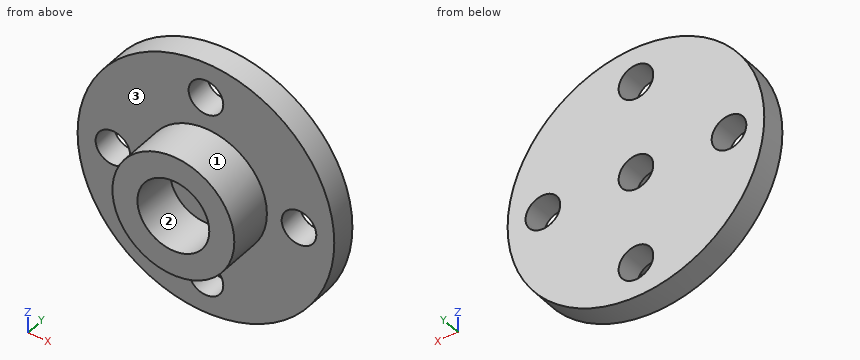
```python
from build123d import *

# Parameters (mm, degrees)
F0_R     = 10
F1_DEPTH = 2
F2_R     = 4.75
F2_R_2   = 2.8
F3_DEPTH = 3.6
F4_R     = 1.35
F5_DEPTH = 25


with BuildPart() as f1:
    # F0 (on Front) → F1 (new body)
    with BuildSketch(Plane.XZ):
        Circle(F0_R)
    extrude(amount=F1_DEPTH)

    # F2 (on face) → F3 (join)
    with BuildSketch(Plane.XZ.offset(2)):
        Circle(F2_R)
        Circle(F2_R_2, mode=Mode.SUBTRACT)
    extrude(amount=F3_DEPTH)

    # F4 (on face) → F5 (cut)
    with BuildSketch(Plane.XZ.offset(2)):
        with Locations((0, 7.25)):
            Circle(F4_R)
        with Locations((-7.25, 0)):
            Circle(F4_R)
        Circle(F4_R)
        with Locations((7.25, 0)):
            Circle(F4_R)
        with Locations((0, -7.25)):
            Circle(F4_R)
    extrude(amount=-F5_DEPTH, mode=Mode.SUBTRACT)


solid = f1.part
```
Source: CAD feature listing. Evaluate the final solid. Frame: model axes, mm. Face numbers are marked on the shaded views. Round coordinates to 2 decimals unless told otherwise and drop trailing zeros. Loops run counter-clockwise (first coordinate to the right, second up) from the corner with the lowest first, then second, coordinate; pieces in that order, holes last. Notation, with made-up numbers: M -2,36 L 20,36 A32 ccw 20,70 Z; hole C -27.75,84.25 d1. An arc over 180 degrees is marked long. Use a Markdown table: item, result. Add a question column.
1. Mould query, pull axis X, two halves, no side actions, for the marked faces 1, 2 and 3. Classes: pulls with the +X half, pulls with the -X half, needs draft (parallel to the pull), parting line crosses it, or undercut.
2. Line query: line 1 (Z direction, x = 0, y = -1.3); line 2 (Z direction, x = 0, y = -4.3); line 3 (Y direction, x = -4.25, z = -3). Output: solid intervals per line, ascending.
3. Section query C-C on z = -7.25. Return the cut outline in (x, y).
4. Section query B-B on y = -0.45. Return the cut outline in (x, z), then the cut area to 3 significant figures.
5. Section query D-D on x = -7.25. Return the cut outline in (y, z).
6. Contact query for flat-ended pins moving along their axis: P1, Ø2, axis at x = 7.25, z = 0, coming from the +Y side; P2, Ø4.5, axis at x = 0, z = 0, coming from the -Y side; P3, Ø3, axis at y = -2.5, z = -3, coming from the +X side; P4, Ø2, axis at y = -2.5, z = 1.5, coming from the -X side. Output: stop coordinate, or through.
7. Section query A-A on z = 0. Return the cut outline in (x, y).
Reported:
| question | item | result |
|---|---|---|
| 1 | face 1 | parting line crosses it |
| 1 | face 2 | undercut |
| 1 | face 3 | needs draft |
| 2 | line 1 | z = -10 to -8.6, -5.9 to -1.35, 1.35 to 5.9, 8.6 to 10 |
| 2 | line 2 | z = -4.75 to -2.8, 2.8 to 4.75 |
| 2 | line 3 | y = -2 to 0 |
| 3 | outline | M -6.89,-2 L -1.35,-2 L -1.35,0 L -6.89,0 Z; M 1.35,-2 L 6.89,-2 L 6.89,0 L 1.35,0 Z |
| 4 | outline | C 0,0 d20; hole C -7.25,0 d2.7; hole C 0,-7.25 d2.7; hole C 0,0 d2.7; hole C 0,7.25 d2.7; hole C 7.25,0 d2.7 |
| 4 | area | 286 mm² |
| 5 | outline | M -2,-6.89 L 0,-6.89 L 0,-1.35 L -2,-1.35 Z; M -2,1.35 L 0,1.35 L 0,6.89 L -2,6.89 Z |
| 6 | P1 | passes through |
| 6 | P2 | stops at y = -2 |
| 6 | P3 | stops at x = 9.87 |
| 6 | P4 | stops at x = -9.98 |
| 7 | outline | M -10,-2 L -8.6,-2 L -8.6,0 L -10,0 Z; M -5.9,-2 L -4.75,-2 L -4.75,-5.6 L -2.8,-5.6 L -2.8,-2 L -1.35,-2 L -1.35,0 L -5.9,0 Z; M 1.35,-2 L 2.8,-2 L 2.8,-5.6 L 4.75,-5.6 L 4.75,-2 L 5.9,-2 L 5.9,0 L 1.35,0 Z; M 8.6,-2 L 10,-2 L 10,0 L 8.6,0 Z |
